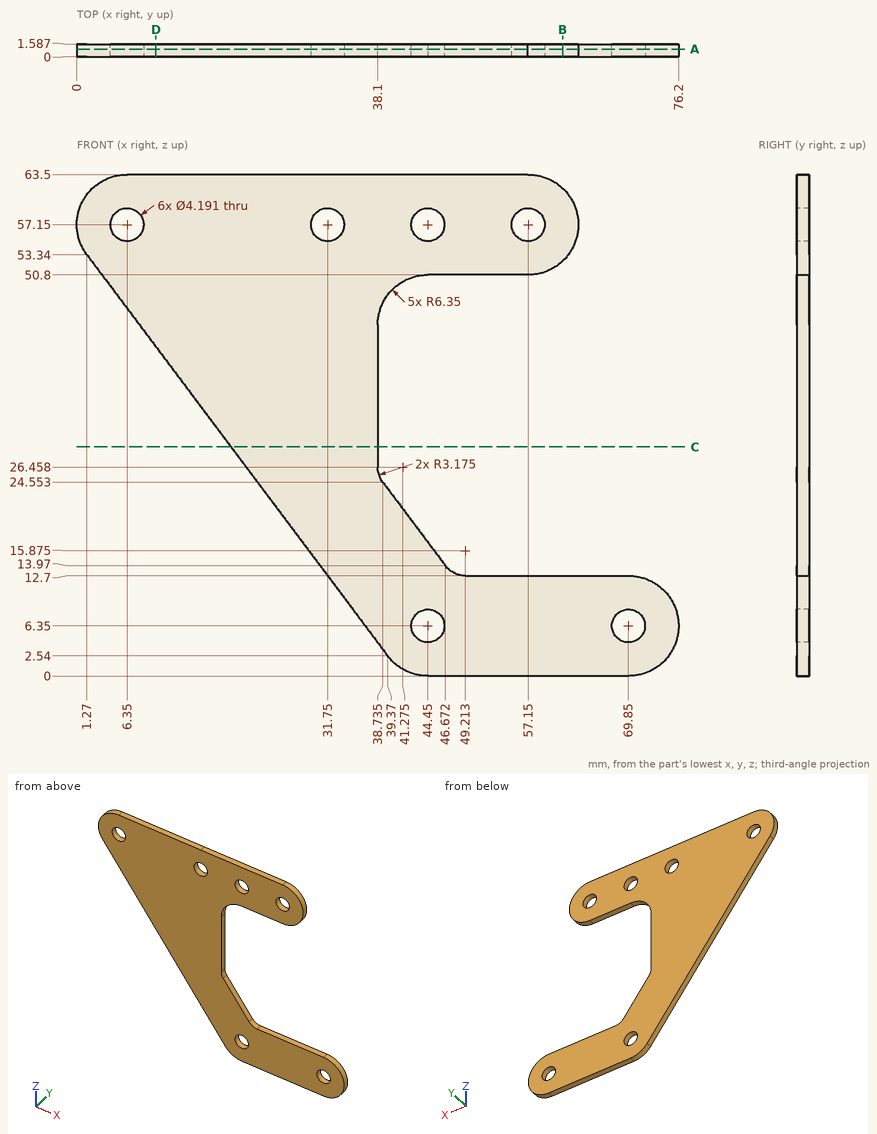
The figure shows three views and two pictorial views of one solid part (mm, origin at its lowest corner). Answer the questions. Give positions to 0.01 mm unless a question says otherwise; leave off trailing zeros. Write each loop counter-clockwise with the first axis right and the second up, starting at its lowest first coordinate (ties: lowest second). Pieces come first, ordered by that corner, then holes. Notation, with made-up numbers: (13.5, 81) -> (68.5, 81) arc R30 cw to (68.5, 120) -> close; hole circle Ø11 at (-30, 61). An arc over 180 degrees is marked (long way). Use one line per item in the form item = value.
1) Section B-B on x = 61.5 is taken. Write down the section's boundary in (y, z).
Result:
outline = (0, 0) -> (1.59, 0) -> (1.59, 12.7) -> (0, 12.7) -> close; (0, 52.52) -> (1.59, 52.52) -> (1.59, 61.78) -> (0, 61.78) -> close
2) Section C-C on z = 29 is taken. Write down the section's boundary in (x, y) (1 decimal).
Result:
outline = (19.5, 0) -> (38.1, 0) -> (38.1, 1.6) -> (19.5, 1.6) -> close
3) Each of these flat-tipped pins is pushed along its axis until it touches: P1, Ø5.5, axis at x = 31.75, z = 57.15, coming from the -Y side; P2, Ø3.5, axis at x = 44.45, z = 57.15, coming from the +Y side. Where does it stop, or does it pass through?
Result:
P1 = 0
P2 = through
4) Section D-D on x = 10 is taken. Write down the section's boundary in (y, z).
Result:
outline = (0, 41.7) -> (1.59, 41.7) -> (1.59, 63.5) -> (0, 63.5) -> close
5) Straight lines are drawn through the part: probe 1 along Z at (x, y) = (70, 0.6); probe 2 along Z at (x, y) = (43.5, 1.3) (1 decimal); probe 3 along Z at (x, y) = (44.45, 1.25) (1 decimal). For each, find the intervals that lie inside material, in ascending order.
Result:
probe_1 = 0 to 4.26, 8.44 to 12.7
probe_2 = 0.1 to 4.5, 8.2 to 18.2, 50.7 to 55.3, 59 to 63.5
probe_3 = 0 to 4.3, 8.4 to 16.9, 50.8 to 55.1, 59.2 to 63.5
6) Section A-A on y = 0.95 is taken. Count the separate pieces of the cut face and the enclosed holes in it, plus the area to 3 significant figures.
Result:
separate_pieces = 1
enclosed_holes = 6
area = 2,030 mm²
